from build123d import *

# Parameters (mm, degrees)
CROQUIS1_W              = 15.961432879
CROQUIS1_H              = 30
SALIENTE_EXTRUIR1_DEPTH = 5.5


with BuildPart() as part:
    # Croquis1 → Saliente-Extruir1 (new body)
    with BuildSketch(Plane(origin=(0, 0, 0), x_dir=(-1, 0, 0), z_dir=(0, 1, 0))):
        Polygon((-73.586706802, 402.295789036), (-73.586706802, 292.295789036), (211.413293198, 292.295789036), (211.413293198, 2.295789036), (-228.586706802, 2.295789036), (-228.586706802, 402.295789036), (-143.586706802, 402.295789036), align=None)
        with Locations((-135.605990362, 360.295789036)):
            Rectangle(CROQUIS1_W, CROQUIS1_H, mode=Mode.SUBTRACT)
    extrude(amount=SALIENTE_EXTRUIR1_DEPTH)


solid = part.part
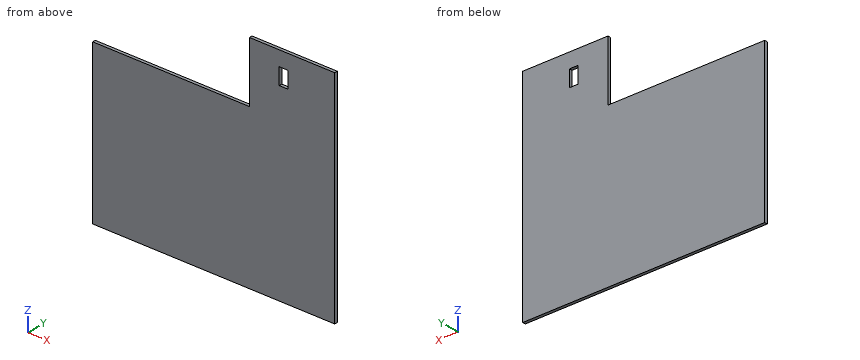
Could you check a few things on this model? Use its own coordinates, in mm. Coordinates: 2 decimals unless noted, no trailing zeros. Loops run counter-clockwise (first coordinate to the right, second up) from the corner with the lowest first, then second, coordinate; pieces in that order, holes last.
1. Imagine slicing it at B-B (z = 299). Please give me the cut outline in (x, y), and give its area (4 significant figures).
2. Imagine slicing it at A-A (y = 3.5). Please give me the cut outline in (x, z).
3. I need wall thicknesses on L1, parallel to X at y = 4.7, z = 355; L2, parallel to Z at x = 41.5, y = 3.45; L3, parallel to X at y = 3.25, z = 307.5. Which ranges of each line are inside material? Lowest first, please.
4. Imagine slicing it at C-C (x = 33). Please give me the cut outline in (y, z).
Computed values:
1. outline: (73.59, 0) - (228.59, 0) - (228.59, 5.5) - (73.59, 5.5) - close
1. area: 852.5 mm2
2. outline: (-211.41, 2.3) - (228.59, 2.3) - (228.59, 402.3) - (73.59, 402.3) - (73.59, 292.3) - (-211.41, 292.3) - close; hole (127.63, 345.3) - (143.59, 345.3) - (143.59, 375.3) - (127.63, 375.3) - close
3. L1: x = 73.59 to 127.63, 143.59 to 228.59
3. L2: z = 2.3 to 292.3
3. L3: x = 73.59 to 228.59
4. outline: (0, 2.3) - (5.5, 2.3) - (5.5, 292.3) - (0, 292.3) - close
